Autodesk Inventor part; units mm, degrees
ref_plane "Work Plane1" through (2.75, 0, 0) normal (0, -1, 0) x (1, 0, 0)
ref_plane "YZ Plane" through (0, 0, 0) normal (1, 0, 0) x (0, 1, 0)
ref_plane "XZ Plane" through (0, 0, 0) normal (0, 1, 0) x (-1, 0, 0)
sketch "Schizzo1" plane through (0, 0, 0) normal (0, 0, 1) x (1, 0, 0)
  line L0 (40, 3) -> (40, 0)
  line L1 (-9, 0) -> (40, 0)
  line L2 (-18.8, 0) -> (49.8, 0)
  line L3 (0, 3.6) -> (0, -0.6)
  line L4 (-9, 3) -> (-9, 0)
  line L5 (22, 3) -> (22, 0) construction
  line L6 (-18.8, 0) -> (49.8, 0)
  line L7 (-9, 3) -> (40, 3)
  dimension "d4" = 9
  dimension "d5" = 40
  dimension "d6" = 18
  dimension "d13" = 6
revolve "Corpo" add sketch "Schizzo1" angle 360 about axis through (-9, 0, 0) along (1, 0, 0)
thread "Filettatura1"
thread "Filettatura2"
chamfer "Smusso1" distance 0.6145 distance2 0.6135 1 edges at (40, -3, 0) measured on face at (40, 1.0659, 1.0214)
chamfer "Smusso2" distance 0.5423 distance2 0.6135 1 edges at (-9, -3, 0) measured on face at (23.2577, 2.9903, -0.2414)
ref_plane "Work Plane1" through (2.75, 0, 0) normal (0, -1, 0) x (1, 0, 0)
equation "\"d4\" = KOH"
equation "\"d5\" = NLG"
equation "\"d6\" = GEL"
equation "\"d13\" = GD"
equation "\"d1\" = KOH"
equation "\"d7\" = GEL + GAL"
equation "\"d10\" = -0.5 * SPD + 0.5 * GD"
equation "\"d12\" = -0.5 * SPD + 0.5 * GD"
equation "\"NLG\" = 40"
equation "\"GEL\" = 18"
equation "\"GAL\" = 0.61345 * PTC"
equation "\"SPD\" = NND - 1.2269 * PTC"
equation "\"d0\" = GD"
equation "\"GUL\" = 0.61345 * PTC"
equation "\"KOH\" = 9"
equation "\"GD\" = NND"
equation "\"BDM\" = NND"
equation "\"GUL1\" = 0.54127"
equation "\"GAL1\" = 1"
equation "\"d80\" = -GUL - GEL"
equation "\"d86\" = -KOH + GUL1"
equation "\"PTC\" = 1"
equation "\"THREADDIA\" = 6"
equation "\"TOA\" = 30deg"
equation "\"NND\" = 6"
equation "\"GD1\" = THREADDIA - 1.2269 * PTC"
properties part number "UNI 5909 - M6 x 40" material "Acciaio, Dolce"
Model file for the job. Use its own axes, mm. Give positions to 0.01 mm unless a question says otherwise; leave off trailing zeros. Write each loop counter-clockwise with the first axis right and the second up, starting at its lowest first coordinate (ties: lowest second). Pieces come first, ordered by that corner, then holes. Notation, with made-up numbers: (-28, 21.25) - (-17, 21.25) arc R16 ccw to (-17, 51.25) - close; hole circle Ø2 at (-35, -0.5). An arc over 180 degrees is marked (long way). One line per question, with ' | ' between items. Start each with the question number.
(1) Wall check: line 1 along Y through (x, z) = (19, -0.25); line 2 along Z through (x, y) = (22.5, 0.1); line 3 along X through (y, z) = (-2.15, -1.3). Give the ranges that are in metal, low to high. Write a range as from..to.
(2) Slice it at A-A on x = 9. Write the cut outline in (y, z), plus the area to 3 significant figures.
(3) Pin check, flat tips, straight feed: P1, Ø1, axis at x = 2.5, y = 2, coming from the -Z side; P2, Ø2, axis at x = 5, y = 2.5, coming from the +Z side; P3, Ø3, axis at x = 0.5, y = 2, coming from the -Z side. Stop position of each tip, or through.
Results below:
1) line 1: -2.99..2.99 | line 2: -3..3 | line 3: -8.89..39.87
2) outline: circle Ø6 at (0, 0) | area: 28.3 mm^2
3) P1: z = -2.6 | P2: z = 2.6 | P3: z = -2.96
